Autodesk Inventor part; units mm, degrees
ref_plane "Start plane" through (0, 0, 40) normal (0, 0, 1) x (1, 0, 0)
ref_plane "End plane" through (0, 0, 611) normal (0, 0, 1) x (1, 0, 0)
ref_plane "Work Plane4" through (7, -310, 40) normal (0, 0, -1) x (-1, 0, 0)
ref_plane "Start plane" through (0, 0, 40) normal (0, 0, 1) x (1, 0, 0)
ref_plane "End plane" through (0, 0, 611) normal (0, 0, 1) x (1, 0, 0)
sketch "Sketch" plane through (0, 0, 0) normal (0, 0, 1) x (1, 0, 0)
  line L0 (-15, -17) -> (-15, 17)
  line L1 (-12, 20) -> (12, 20)
  line L2 (15, 17) -> (15, -17)
  line L3 (12, -20) -> (-12, -20)
  arc A0 (-15, -17) -> (-12, -20) centre (-12, -17) ccw
  arc A1 (-12, 20) -> (-15, 17) centre (-12, 17) ccw
  arc A2 (15, 17) -> (12, 20) centre (12, 17) ccw
  arc A3 (12, -20) -> (15, -17) centre (12, -17) ccw
  arc A4 (-12, 18) -> (-13, 17) centre (-12, 17) ccw
  line L4 (-12, 18) -> (12, 18)
  arc A5 (13, 17) -> (12, 18) centre (12, 17) ccw
  line L5 (13, 17) -> (13, -17)
  arc A6 (12, -18) -> (13, -17) centre (12, -17) ccw
  line L6 (12, -18) -> (-12, -18)
  arc A7 (-13, -17) -> (-12, -18) centre (-12, -17) ccw
  line L7 (-13, -17) -> (-13, 17)
  line L8 (0, 28.8698) -> (0, -28.8698) construction
  line L9 (-14.8698, 0) -> (14.8698, 0) construction
  dimension "d7" = 3
  dimension "d10" = 40
  dimension "d11" = 30
  dimension "d12" = 2
  dimension "d15" = 20
  dimension "d16" = 15
extrude "Body" add sketch "Sketch" along normal up to surface (571 mm away) from surface at 40
sketch "Sketch3" plane through (0, 0, 0) normal (0, 0, 1) x (1, 0, 0)
  line L0 (0, 0) -> (10, 0)
ref_plane "Work Plane3" through (0, 0, 0) normal (0, -1, 0) x (1, 0, 0)
sketch "Sketch4" plane through (0, 0, 0) normal (0, -1, 0) x (1, 0, 0)
  line L0 (-2, 40) -> (12, 40)
  line L1 (-2, 611) -> (12, 611)
  dimension "d18" = 571
ref_plane "Work Plane4" through (7, -310, 40) normal (0, 0, -1) x (-1, 0, 0)
split "Split1" plane through (7, -310, 40) removes the side toward (0, 0, -1)
ref_plane "Work Plane5" through (-37, -100, 611) normal (0, 0, 1) x (1, 0, 0)
split "Split2" plane through (-37, -100, 611) removes the side toward (0, 0, 1)
equation "\"d7\" = G_IR"
equation "\"d10\" = G_H"
equation "\"d11\" = G_W"
equation "\"d12\" = G_T"
equation "\"d15\" = 0.5 * d10"
equation "\"d16\" = 0.5 * d11"
equation "\"d3\" = G_L"
equation "\"G_W\" = 30"
equation "\"G_H\" = 40"
equation "\"G_T\" = 2"
equation "\"G_IR\" = 3"
equation "\"G_L\" = d18"
equation "\"G_OFFSET_START\" = -40"
equation "\"G_OFFSET_END\" = -40"
equation "\"d13\" = -G_OFFSET_START"
equation "\"d14\" = G_OFFSET_END + B_L"
equation "\"B_L\" = 651"
properties part number "UNI EN 10305-5 - 40 x 30 x 2  - 571" material "Steel, Mild"
Source: CAD feature listing. Evaluate the final solid. Frame: model axes, mm. A direction names the side the tool comes from. Coordinates: 2 decimals unless noted, no trailing zeros. Write each loop counter-clockwise with the first axis right and the second up, starting at its lowest first coordinate (ties: lowest second). Pieces come first, ordered by that corner, then holes. Notation, with made-up numbers: (73, -4) -> (132, -4) arc R33 ccw to (132, 29) -> close; hole circle Ø5 at (27.5, 2). An arc over 180 degrees is marked (long way). Return JSON: item names as keys, results as strings. Group by question number.
1) Section query A-A, the plane z = 278.5. Return loops of the section in (x, y).
2) Mould query, pull axis Y, two halves, no side actions, for faces 1 (the face through (0, 18, 322)), 2 (the face through (-15, 0, 322)), 3 (the face through (0, 20, 322)). Classes: +Y half, -Y half, draft (parallel to the pull), parting line (faces both ways), or undercut.
3) Section query B-B, the plane y = -11.5. Return loops of the section in (x, z).
4) Section query C-C, the plane x = -3. Return loops of the section in (y, z).
5) Set-up query: faces 4 (the face through (15, 0, 322)), 5 (the face through (0, -18, 322)). Return all of +Z, -Z, +X, -X, +Y, -Y with unobstructed straight access to the full face (end or side cutting, diameter ignored); none if empty.
6) Ray query, line 1 along Y through (x, z) = (-4.25, 86.5); line 2 along X through (y, z) = (4, 512); line 3 along Y through (x, z) = (-13.75, 485). Return the intervals inside material, ascending.
From the geometry:
{
 "1": {"outline": "(-15, -17) arc R3 ccw to (-12, -20) -> (12, -20) arc R3 ccw to (15, -17) -> (15, 17) arc R3 ccw to (12, 20) -> (-12, 20) arc R3 ccw to (-15, 17) -> close; hole (-13, -17) arc R1 ccw to (-12, -18) -> (12, -18) arc R1 ccw to (13, -17) -> (13, 17) arc R1 ccw to (12, 18) -> (-12, 18) arc R1 ccw to (-13, 17) -> close"},
 "2": {"face 1": "undercut", "face 2": "draft", "face 3": "+Y half"},
 "3": {"outline": "(-15, 40) -> (-13, 40) -> (-13, 611) -> (-15, 611) -> close; (13, 40) -> (15, 40) -> (15, 611) -> (13, 611) -> close"},
 "4": {"outline": "(-20, 40) -> (-18, 40) -> (-18, 611) -> (-20, 611) -> close; (18, 40) -> (20, 40) -> (20, 611) -> (18, 611) -> close"},
 "5": {"face 4": "+Z, -Z, +X, +Y, -Y", "face 5": "+Z, -Z"},
 "6": {"line 1": "-20 to -18, 18 to 20", "line 2": "-15 to -13, 13 to 15", "line 3": "-19.44 to 19.44"}
}
